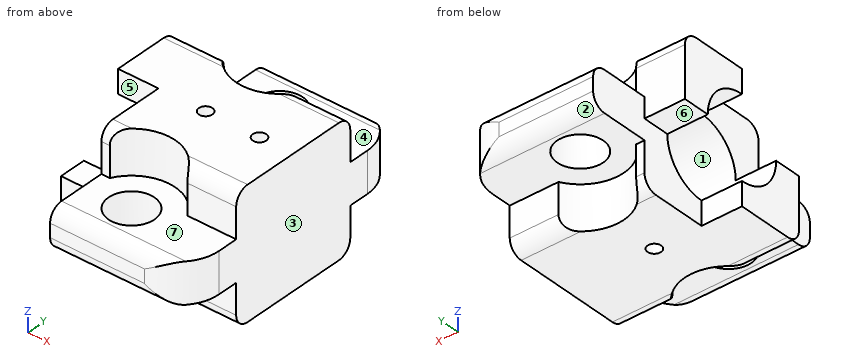
Autodesk Inventor part; units mm, degrees
ref_plane "YZ Plane" through (0, 0, 0) normal (1, 0, 0) x (0, 1, 0)
ref_plane "XZ Plane" through (0, 0, 0) normal (0, 1, 0) x (-1, 0, 0)
ref_plane "XY Plane" through (0, 0, 0) normal (0, 0, 1) x (1, 0, 0)
sketch "Skizze3" plane through (0, 0, 0) normal (1, 0, 0) x (0, 1, 0)
  line L0 (4, 9.5) -> (-4, 9.5)
  line L1 (-5, 8.5) -> (-5, 1)
  line L2 (-4, 0) -> (4, 0)
  line L3 (5, 1) -> (5, 8.5)
  arc A0 (5, 8.5) -> (4, 9.5) centre (4, 8.5) ccw
  arc A1 (-4, 9.5) -> (-5, 8.5) centre (-4, 8.5) ccw
  arc A2 (-5, 1) -> (-4, 0) centre (-4, 1) ccw
  arc A3 (4, 0) -> (5, 1) centre (4, 1) ccw
  line L4 (-5, 6.25) -> (-9.5, 6.25)
  line L5 (-9.5, 6.25) -> (-9.5, 3.25)
  line L6 (-9.5, 3.25) -> (-5, 3.25)
  line L7 (5, 6.25) -> (9.5, 6.25)
  line L8 (9.5, 6.25) -> (9.5, 3.25)
  line L9 (9.5, 3.25) -> (5, 3.25)
  point P0 (-5, 0)
  point P1 (-5, 9.5)
  point P2 (5, 0)
  point P3 (0, 0)
  point P4 (0, 0)
  point P5 (-9.5, 4.75)
  point P6 (-5, 4.75)
  point P7 (9.5, 4.75)
  point P8 (5, 4.75)
  dimension "d12" = 10
  dimension "d13" = 9.5
  dimension "d14" = 1
  dimension "d83" = 4.5
  dimension "d84" = 3
extrude "Extrusion3" add sketch "Skizze3" along normal blind 10 and the other way blind 3 contours A0 L3 A3 L2 A2 L1 A1 L0
extrude "Extrusion4" add sketch "Skizze3" along normal blind 10 and the other way blind 3 contours L7 L8 L9 L3 | L1 L6 L5 L4
fillet "Rundung1" radius 3 4 edges at (-3, -9.5, 4.75) (10, -9.5, 4.75) (10, 9.5, 4.75) (-3, 9.5, 4.75)
sketch "Skizze5" plane through (-3, 0, 0) normal (-1, 0, 0) x (0, 0, 1)
  line L0 (1, -5) -> (8.5, -5)
  line L1 (9.5, -4) -> (9.5, 4)
  point P0 (0, 0)
  point P1 (4.75, 0)
  point P2 (4.75, -5)
  point P3 (9.5, 0)
hole "Bohrung3" at (-3, 0, 4.75) direction (1, 0, 0) diameter 6 depth 12
sketch "Skizze6" plane through (-3, -4, 9.5) normal (0, 0, 1) x (1, 0, 0)
  line L0 (0, 0) -> (0, 8)
  point P0 (3, 4)
  point P1 (3, 4)
  point P2 (0, 8)
  point P3 (0, 4)
  point P4 (0, 4)
  dimension "d41" = 3
sketch "Skizze7" plane through (-3, -4, 9.5) normal (0, 0, 1) x (1, 0, 0)
  line L0 (13, 8) -> (13, 0)
  line L1 (0, 0) -> (0, 8)
  line L2 (12, 7) -> (12, 1)
  point P0 (6.5, 4)
  point P1 (13, 4)
  dimension "d122" = 5.5
hole "Bohrung5" at (3.5, 0, 9.5) direction (0, 0, -1) diameter 1 end through all
sketch "Skizze9" plane through (0, -5, 6.25) normal (0, 0, 1) x (1, 0, 0)
  arc A0 (-3, -1.5) -> (0, -4.5) centre (0, -1.5) ccw
  line L0 (-3, 0) -> (10, 0)
  arc A1 (0, 14.5) -> (-3, 11.5) centre (0, 11.5) ccw
  line L1 (10, 10) -> (-3, 10)
  line L2 (-3, 10) -> (-3, 11.5)
  line L3 (10, 11.5) -> (10, 10)
  line L4 (10, 0) -> (10, -1.5)
  line L5 (-3, -1.5) -> (-3, 0)
  arc A2 (10, 11.5) -> (7, 14.5) centre (7, 11.5) ccw
  line L6 (7, 14.5) -> (0, 14.5)
  line L7 (0, -4.5) -> (7, -4.5)
  arc A3 (7, -4.5) -> (10, -1.5) centre (7, -1.5) ccw
  point P0 (0, 5)
  point P1 (3.5, -1.5)
  point P2 (3.5, 11.5)
  point P3 (3.5, 14.5)
  point P4 (3.5, -4.5)
hole "Bohrung6" at (3.5, 6.5, 6.25) at (3.5, -6.5, 6.25) direction (0, 0, -1) diameter 3.4 end through all
hole "Bohrung7" at (3.5, -6.5, 6.25) at (3.5, 6.5, 6.25) direction (0, 0, 1) diameter 3.4 end through all counterbore diameter 6.5 counterbore depth 3.4
sketch "Skizze10" plane through (10, -5, 3.25) normal (0, 0, -1) x (-1, 0, 0)
  arc A0 (5.7, 0) -> (7.3, 0) centre (6.5, -1.5) ccw
  arc A1 (7.3, 10) -> (5.7, 10) centre (6.5, 11.5) ccw
  point P0 (10, 5)
hole "Bohrung8" at (3.5, -6.5, 3.25) at (3.5, 6.5, 3.25) direction (0, 0, -1) diameter 3.4 end through all counterbore diameter 6.5 counterbore depth 3.4
sketch "Skizze11" plane through (-3, 0, 0) normal (-1, 0, 0) x (0, 0, 1)
  circle A0 centre (4.75, 0) radius 3
  line L0 (3.25, 6.5) -> (6.25, 6.5)
  line L1 (3.25, 6.5) -> (3.25, 5)
  line L2 (3.25, 5) -> (1, 5)
  arc A1 (1, 5) -> (0, 4) centre (1, 4) ccw
  line L3 (0, 4) -> (0, -4)
  arc A2 (0, -4) -> (1, -5) centre (1, -4) ccw
  line L4 (1, -5) -> (3.25, -5)
  line L5 (3.25, -5) -> (3.25, -6.5)
  line L6 (6.25, -6.5) -> (3.25, -6.5)
  line L7 (6.25, -6.5) -> (6.25, -5)
  line L8 (6.25, -5) -> (8.5, -5)
  arc A3 (8.5, -5) -> (9.5, -4) centre (8.5, -4) ccw
  line L9 (9.5, -4) -> (9.5, 4)
  arc A4 (9.5, 4) -> (8.5, 5) centre (8.5, 4) ccw
  line L10 (8.5, 5) -> (6.25, 5)
  line L11 (6.25, 5) -> (6.25, 6.5)
  line L12 (6.25, 5) -> (3.25, 5)
  line L13 (0.4, 4.8) -> (9.1, 4.8)
  line L14 (6.25, -3.25) -> (6.25, -5)
  line L15 (6.25, -5) -> (3.25, -5)
  line L16 (0.4, -4.8) -> (9.1, -4.8)
  line L17 (9.5, -4) -> (9.5, 4)
  line L18 (9.5, 0) -> (0, 0)
  line L19 (3.25, 9.5) -> (3.25, 6.5)
  line L20 (3.25, 6.5) -> (6.25, 6.5)
  line L21 (6.25, 6.5) -> (6.25, 9.5)
  line L22 (6.25, 9.5) -> (3.25, 9.5)
  line L23 (6.25, -9.5) -> (6.25, -6.5)
  line L24 (6.25, -6.5) -> (3.25, -6.5)
  line L25 (3.25, -6.5) -> (3.25, -9.5)
  line L26 (3.25, -9.5) -> (6.25, -9.5)
  line L27 (4.75, 5) -> (4.75, -5)
  point P0 (9.1757, 4.7372)
  point P1 (0.3243, -4.7372)
  point P2 (1.75, 0)
  point P3 (7.75, 0)
  point P4 (4.75, 3)
  point P5 (4.75, -3)
extrude "Extrusion7" cut sketch "Skizze11" against normal blind 3 contours L18 L27 A0 | L18 L9 A3 L16 L27 A0 | A0 L27 L18 | L27 L18 A0 | A0 L18 L3 A1 L13 L27 | A0 L18 L27 | L13 A1 L2 L12 L27 | L16 L14 L15 L27 | L12 L1 L0 L11 | L16 A3 L8 L14 | L15 L7 L6 L5 | L0 L19 L22 L21 | L23 L26 L25 L6
sketch "Skizze12" plane through (-3, 4, 9.5) normal (0, 0, 1) x (1, 0, 0)
  line L0 (12, -1) -> (12, -7)
  point P0 (3, -4)
  point P1 (10.5, -4)
  point P2 (12, -4)
  dimension "d113" = 1.5
hole "Bohrung9" at (7.5, 0, 9.5) direction (0, 0, -1) diameter 1 depth 3.25
sketch "Skizze13" plane through (0, 0, 0) normal (-1, 0, 0) x (0, 0, 1)
  line L0 (3.25, 9.5) -> (6.25, 9.5)
  line L1 (5.25, 9.5) -> (4.25, 9.5)
  line L2 (3.25, 8.5) -> (3.25, 5)
  line L3 (6.25, 8.5) -> (6.25, 5)
  line L4 (6.25, -5) -> (6.25, -8.5)
  line L5 (3.25, -9.5) -> (6.25, -9.5)
  line L6 (5.25, -9.5) -> (4.25, -9.5)
  line L7 (3.25, -8.5) -> (3.25, -5)
  line L8 (3.25, -8.2) -> (3.25, -4.8)
  arc A0 (6.25, 8.5) -> (5.25, 9.5) centre (5.25, 8.5) ccw
  arc A1 (4.25, 9.5) -> (3.25, 8.5) centre (4.25, 8.5) ccw
  arc A2 (3.25, -8.5) -> (4.25, -9.5) centre (4.25, -8.5) ccw
  arc A3 (5.25, -9.5) -> (6.25, -8.5) centre (5.25, -8.5) ccw
  line L9 (6.25, 9.5) -> (6.25, 5)
  line L10 (3.25, 5) -> (3.25, 9.5)
  line L11 (6.25, -5) -> (6.25, -9.5)
  line L12 (3.25, -9.5) -> (3.25, -5)
  point P0 (0, 0)
  point P1 (5.25, 9.5)
  point P2 (4.25, 9.5)
  dimension "d123" = 1
extrude "Extrusion8" cut sketch "Skizze13" against normal through all
properties part number "BT015_huenin20_23" material "E360"
Could you check a few things on this model? Use its own coordinates, in mm. Face numbers are marked on the shaded views. A direction names the side the tool comes from. Give positions to 0.01 mm unless a question says otherwise; leave off trailing zeros. Order: outer loops, then holes, each group sorted by start corner. A loop starts at its lowest first (then second) coordinate and runs counter-clockwise, first axis right, second up. Notation, with made-up numbers: (82, 88) -> (122, 88) arc R23 ccw to (122, 107) -> close; hole circle Ø6 at (53.5, 72.25). An arc over 180 degrees is marked (long way). Return JSON: item names as keys, results as strings.
1. Imagine slicing it at D-D on x = 5. List the corners of the cut face in (y, z) for me.
Answer list:
{"outline": "(-9.5, 4.25) arc R1 ccw to (-8.5, 3.25) -> (-7.3, 3.25) -> (-7.3, 6.25) -> (-8.5, 6.25) arc R1 ccw to (-9.5, 5.25) -> close; (-5.7, 3.25) -> (-3.62, 3.25) -> (-3.62, 0) -> (3.62, 0) -> (3.62, 3.25) -> (5.7, 3.25) -> (5.7, 6.25) -> (3.62, 6.25) -> (3.62, 9.5) -> (-3.62, 9.5) -> (-3.62, 6.25) -> (-5.7, 6.25) -> close; (7.3, 3.25) -> (8.5, 3.25) arc R1 ccw to (9.5, 4.25) -> (9.5, 5.25) arc R1 ccw to (8.5, 6.25) -> (7.3, 6.25) -> close; hole circle Ø6 at (0, 4.75)"}
2. Imagine slicing it at A-A on x = -1.25. List the corners of the cut face in (y, z) for me.
Answer list:
{"outline": "(-5, 1) arc R1 ccw to (-4, 0) -> (0, 0) -> (0, 1.75) arc R3 cw to (-3, 4.75) -> (-5, 4.75) -> close; (0, 7.75) arc R3 cw to (3, 4.75) -> (5, 4.75) -> (5, 8.5) arc R1 ccw to (4, 9.5) -> (0, 9.5) -> close"}
3. Imagine slicing it at B-B on x = 3.5. Give the number of separate pieces and of enclosed holes in the cut face, then the cut area to 3 significant figures.
Answer list:
{"separate pieces": "4", "enclosed holes": "0", "area": "46.2 mm2"}
4. Imagine slicing it at C-C on y = -1. List the corners of the cut face in (x, z) for me, then the cut area to 3 significant figures.
Answer list:
{"outline": "(-3, 0) -> (10, 0) -> (10, 9.5) -> (0, 9.5) -> (0, 7.58) -> (9, 7.58) -> (9, 1.92) -> (-3, 1.92) -> close", "area": "49.9 mm2"}
5. I need wall thicknesses on line 1 (Y direction, x = 1, z = 4.75); line 2 (Y direction, x = 3.5, z = 4.55); line 3 (Y direction, x = 3.5, z = 0.4). Which ranges of each line are inside material? Lowest first, please. Write a range as from..to.
Answer list:
{"line 1": "y = -9.5..-3, 3..9.5", "line 2": "y = -9.5..-8.2, -4.8..-2.99, 2.99..4.8, 8.2..9.5", "line 3": "y = -3.25..-0.5, 0.5..3.25"}
6. For pin 1 Ø5.5 at (x, y) = (3.5, -6.5) entering from +Z; pin 2 Ø1.9 at (y, z) = (4.5, 3) entering from -X; pin 3 Ø1.6 at (x, y) = (-1, 3.5) entering from -Z, each with a flat end and sliding along its axis, tell me the tip position at first contact or that it passes through.
Answer list:
{"pin 1": "stops at z = 6.25", "pin 2": "stops at x = 0", "pin 3": "stops at z = 4.75"}
7. On a 3-axis mill with a long thin cutter (end or side, diameter ignored), from which of +Z, -Z, +X, -X, +Y, -Y can I reach the whole of each face in a straight line? I mean the marked faces 4, 5, 6 and 7. Say none if no direction works.
Answer list:
{"face 4": "+Z, +Y", "face 5": "+Z, -X, -Y", "face 6": "-Z, -X, +Y", "face 7": "+Z, -Y"}
8. Thinking about a two-plate mould opening in Z: for the marked faces 1, 2 and 3, which applies, pulls with the +Z half, pulls with the -Z half, needs draft (parallel to the pull), parting line crosses it, or undercut?
Answer list:
{"face 1": "undercut", "face 2": "pulls with the -Z half", "face 3": "needs draft"}
